Autodesk Inventor part; units mm, degrees
ref_plane "YZ Plane" through (0, 0, 0) normal (1, 0, 0) x (0, 1, 0)
ref_plane "XZ Plane" through (0, 0, 0) normal (0, 1, 0) x (-1, 0, 0)
ref_plane "XY Plane" through (0, 0, 0) normal (0, 0, 1) x (1, 0, 0)
sketch "Sketch1" plane through (0, 0, 0) normal (0, 0, 1) x (1, 0, 0)
  line L0 (-10.4918, 19.8361) -> (-50.4918, 19.8361)
  line L1 (-50.4918, 19.8361) -> (-50.4918, -15.1639)
  line L2 (-50.4918, -15.1639) -> (-10.4918, -15.1639)
  line L3 (-10.4918, -15.1639) -> (-10.4918, 19.8361)
  point P0 (0, 0)
  dimension "d0" = 40
  dimension "d1" = 35
extrude "Extrusion1" add sketch "Sketch1" along normal blind 5
sketch "Sketch2" plane through (0, 0, 0) normal (0, 0, -1) x (-1, 0, 0)
  line L0 (50.4918, 19.8361) -> (50.4918, -15.1639)
  line L1 (50.4918, 19.8361) -> (27.4918, 19.8361)
  line L2 (27.4918, 19.8361) -> (27.4918, 14.8361)
  line L3 (27.4918, 14.8361) -> (50.4918, 14.8361)
  line L4 (50.4918, 14.8361) -> (50.4918, 19.8361)
  point P0 (0, 0)
  point P1 (50.4918, 14.8361)
  dimension "d4" = 23
  dimension "d5" = 5
extrude "Extrusion2" add sketch "Sketch2" along normal blind 20
sketch "Sketch3" plane through (0, 0, 0) normal (0, 0, -1) x (-1, 0, 0)
  line L0 (27.4918, 14.8361) -> (50.4918, 14.8361)
  line L1 (50.4918, 19.8361) -> (50.4918, -15.1639)
  line L2 (50.4918, 15.8361) -> (47.4918, 15.8361)
  line L3 (47.4918, 15.8361) -> (47.4918, -4.1639)
  line L4 (47.4918, -4.1639) -> (50.4918, -4.1639)
  line L5 (50.4918, -4.1639) -> (50.4918, 15.8361)
  point P0 (0, 0)
  point P1 (47.4918, 14.8361)
  dimension "d8" = 20
  dimension "d9" = 3
extrude "Extrusion3" add sketch "Sketch3" along normal blind 20 contours L0 L1 L4 L3
sketch "Sketch4" plane through (-27.4918, 14.8361, -20) normal (0, -1, 0) x (1, 0, 0)
  circle A0 centre (-10, 10) radius 8
  line L0 (0, 0) -> (-20, 0)
  line L1 (0, 20) -> (0, 0)
  circle A1 centre (-2, 2) radius 1
  circle A2 centre (-18, 2) radius 1
  circle A3 centre (-18, 18) radius 1
  circle A4 centre (-2, 18) radius 1
  point P0 (27.4918, 20)
  dimension "d12" = 16
  dimension "d13" = 10
  dimension "d14" = 10
  dimension "d15" = 2
  dimension "d16" = 2
  dimension "d17" = 2
  dimension "d18" = 2
  dimension "d19" = 8
  dimension "d20" = 8
  dimension "d21" = 8
  dimension "d22" = 8
  dimension "d23" = 8
  dimension "d24" = 8
  dimension "d25" = 8
  dimension "d26" = 8
extrude "Extrusion4" cut sketch "Sketch4" against normal through all
fillet "Fillet1" radius 1.5 1 edges at (-27.4918, 17.3361, -20)
sketch "Sketch5" plane through (-47.4918, -4.1639, 0) normal (1, 0, 0) x (0, 0, -1)
  line L0 (20, 19) -> (20, 0)
  line L1 (0, 0) -> (20, 0)
  line L2 (20, 19) -> (0, 0)
  line L3 (0, 0) -> (20, 0)
  line L4 (20, 0) -> (20, 19)
  point P0 (0, 4.1639)
extrude "Extrusion5" cut sketch "Sketch5" against normal through all
fillet "Fillet2" radius 5 1 edges at (-48.9918, -4.1639, 0)
fillet "Fillet4" radius 2 1 edges at (-47.4918, 5.3361, 0)
sketch "Sketch6" plane through (0, 0, 5) normal (0, 0, 1) x (1, 0, 0)
  line L0 (-10.4918, 19.8361) -> (-50.4918, 19.8361)
  line L1 (-17.4918, 19.8361) -> (-43.4918, 19.8361)
  line L2 (-43.4918, 19.8361) -> (-43.4918, 14.8361)
  line L3 (-43.4918, 14.8361) -> (-17.4918, 14.8361)
  line L4 (-17.4918, 14.8361) -> (-17.4918, 19.8361)
  line L5 (-10.4918, -15.1639) -> (-10.4918, 19.8361)
  line L6 (-50.4918, 19.8361) -> (-50.4918, -15.1639)
  point P0 (0, 0)
  dimension "d39" = 5
  dimension "d40" = 7
  dimension "d41" = 7
extrude "Extrusion6" add sketch "Sketch6" along normal blind 46
chamfer "Chamfer2" distance 7 angle 45 2 edges at (-17.4918, 17.3361, 5) (-43.4918, 17.3361, 5)
sketch "Sketch7" plane through (-43.4918, 14.8361, 51) normal (0, -1, 0) x (1, 0, 0)
  circle A0 centre (13, -30.5) radius 1.5
  line L0 (-7, -46) -> (33, -46)
  line L1 (26, -39) -> (26, 0)
  point P0 (43.4918, -51)
  dimension "d47" = 3
  dimension "d48" = 15.5
  dimension "d49" = 13
extrude "Extrusion7" cut sketch "Sketch7" against normal through all
chamfer "Chamfer3" distance 1.8 angle 45 1 edges at (-31.9918, 19.8361, 20.5)
sketch "Sketch8" plane through (-27.4918, 19.8361, 0) normal (0, 1, 0) x (1, 0, 0)
  circle A0 centre (14, -2.5) radius 0.8
  circle A1 centre (6, -2.5) radius 0.8
  line L0 (17, 0) -> (0, 0)
  line L1 (17, 0) -> (17, -5)
  point P0 (27.4918, 0)
  dimension "d55" = 1.6
  dimension "d56" = 1.6
  dimension "d57" = 2.5
  dimension "d58" = 2.5
  dimension "d59" = 3
  dimension "d60" = 8
extrude "Extrusion8" cut sketch "Sketch8" against normal blind 10
chamfer "Chamfer4" distance 0.8 angle 45 2 edges at (-14.2918, 9.8361, 2.5) (-22.2918, 9.8361, 2.5)
fillet "Fillet5" radius 1 2 edges at (-14.2918, 10.6356, 2.5) (-22.2918, 10.6356, 2.5)
sketch "Sketch9" plane through (-50.4918, -15.1639, 0) normal (0, -1, 0) x (1, 0, 0)
  line L0 (40, 0) -> (40, 5)
  line L1 (40, 0) -> (23, 0)
  line L2 (40, 5) -> (26, 5)
  line L3 (26, 5) -> (26, 0)
  line L4 (26, 0) -> (40, 0)
  line L5 (40, 0) -> (40, 5)
  point P0 (50.4918, 0)
  dimension "d67" = 14
extrude "Extrusion9" add sketch "Sketch9" along normal blind 15
sketch "Sketch10" plane through (0, 0, 0) normal (0, 0, -1) x (-1, 0, 0)
  circle A0 centre (17.4918, -25.1639) radius 0.8
  line L0 (10.4918, 19.8361) -> (10.4918, -30.1639)
  line L1 (24.4918, -30.1639) -> (10.4918, -30.1639)
  circle A1 centre (17.4918, -5.1639) radius 0.8
  circle A2 centre (17.4918, 14.8361) radius 0.8
  point P0 (0, 0)
  dimension "d70" = 1.6
  dimension "d71" = 7
  dimension "d72" = 5
  dimension "d75" = 20
extrude "Extrusion10" cut sketch "Sketch10" against normal through all
fillet "Fillet6" radius 3 2 edges at (-50.4918, -15.1639, 2.5) (-24.4918, -15.1639, 2.5)
sketch "Sketch11" plane through (0, 0, 0) normal (0, 0, -1) x (-1, 0, 0)
  circle A0 centre (38.4918, -10.1639) radius 1.5
  circle A1 centre (30.4918, -10.1639) radius 1.5
  circle A2 centre (30.4918, -1.1639) radius 1.5
  circle A3 centre (38.4918, -1.1639) radius 1.5
  circle A4 centre (38.4918, 7.8361) radius 1.5
  circle A5 centre (30.4918, 7.8361) radius 1.5
  line L0 (47.4918, -15.1639) -> (27.4918, -15.1639)
  line L1 (50.4918, -6.3105) -> (50.4918, -12.1639)
  circle A6 centre (22.4918, -10.1639) radius 1.5
  circle A7 centre (22.4918, -1.1639) radius 1.5
  circle A8 centre (22.4918, 7.8361) radius 1.5
  point P0 (0, 0)
  point P1 (37.4918, -15.1639)
  dimension "d89" = 3
  dimension "d90" = 3
  dimension "d91" = 3
  dimension "d92" = 3
  dimension "d93" = 3
  dimension "d94" = 3
  dimension "d95" = 5
  dimension "d96" = 5
  dimension "d97" = 8
  dimension "d98" = 12
  dimension "d99" = 12
  dimension "d100" = 12
  dimension "d101" = 9
  dimension "d102" = 9
  dimension "d103" = 9
  dimension "d104" = 8
  dimension "d105" = 9
  dimension "d106" = 8
  dimension "d109" = 8
  dimension "d110" = 3
  dimension "d111" = 5
  dimension "d112" = 9
  dimension "d113" = 9
  dimension "d114" = 3
  dimension "d115" = 3
  dimension "d116" = 8
  dimension "d117" = 8
extrude "Extrusion11" cut sketch "Sketch11" against normal through all
chamfer "Chamfer7" distance 1.9 angle 45 9 edges at (-20.9918, 7.8361, 0) (-20.9918, -1.1639, 0) (-20.9918, -10.1639, 0) (-28.9918, -10.1639, 0) (-28.9918, -1.1639, 0) (-28.9918, 7.8361, 0) (-36.9918, 7.8361, 0) (-36.9918, -1.1639, 0) (-36.9918, -10.1639, 0)
sketch "Sketch12" plane through (-27.4918, 19.8361, 0) normal (0, 1, 0) x (1, 0, 0)
  circle A0 centre (2, -34) radius 1.5
  circle A1 centre (2, -47) radius 1.5
  circle A2 centre (-9, -34) radius 1.5
  circle A3 centre (-9, -47) radius 1.5
  line L0 (10, -51) -> (-16, -51)
  line L1 (10, -12) -> (10, -51)
  line L2 (-16, -12) -> (-16, -51)
  point P0 (27.4918, 0)
  dimension "d121" = 3
  dimension "d122" = 3
  dimension "d123" = 3
  dimension "d124" = 3
  dimension "d125" = 17
  dimension "d126" = 17
  dimension "d127" = 8
  dimension "d128" = 8
  dimension "d129" = 7
  dimension "d130" = 7
  dimension "d131" = 4
  dimension "d132" = 4
extrude "Extrusion12" cut sketch "Sketch12" against normal through all
fillet "Fillet7" radius 3 1 edges at (-27.4918, 17.3361, 0)
properties part number "Motor_holder_R" material "ABS Plastic"
The listing builds one solid part. Answer for the finished solid, in the listing's coordinates (mm). A direction names the side the tool comes from. Give positions to 0.01 mm unless a question says otherwise; leave off trailing zeros. Order: outer loops, then holes, each group sorted by start corner. A loop starts at its lowest first (then second) coordinate and runs counter-clockwise, first axis right, second up. Notation, with made-up numbers: (-35, 44.5) - (6, 44.5) arc R26 cw to (6, 77.5) - close; hole circle Ø9 at (57, 56.5). An arc over 180 degrees is marked (long way). Answer as CSV lines item,"result".
Q1. A cutting plane is placed at A-A, the plane z = 20.5. Determine the outline of the cut face in (x, y), and give its area (3 significant figures).
Answer key:
outline,"(-43.49, 14.84) - (-31.99, 14.84) - (-31.99, 18.04) - (-33.79, 19.84) - (-43.49, 19.84) - close; (-28.99, 14.84) - (-18.29, 14.84) arc R0.8 cw to (-17.49, 15.64) - (-17.49, 19.84) - (-27.19, 19.84) - (-28.99, 18.04) - close"
area,"111 mm^2"
Q2. A cutting plane is placed at C-C, the plane y = 3.5. Determine the outline of the cut face in (x, z).
Answer key:
outline,"(-50.49, -8.07) - (-47.49, -8.07) - (-47.49, -2) arc R2 cw to (-45.49, 0) - (-10.49, 0) - (-10.49, 5) - (-50.49, 5) - close"
Q3. Each of these flat-tipped pins is pushed along its axis until it touches: pin 1 Ø3.5 at (x, y) = (-38.49, -1.16) entering from +Z; pin 2 Ø12 at (x, y) = (-22.5, -8.5) entering from -Z; pin 3 Ø3 at (x, z) = (-13, 7.5) entering from -Y; pin 4 Ø12 at (x, z) = (-17, 23) entering from +Y. Where does it stop, or does it pass through?
Answer key:
pin 1,"stops at z = 5"
pin 2,"stops at z = 0"
pin 3,"stops at y = 14.84"
pin 4,"stops at y = 19.84"
Q4. A cutting plane is placed at D-D, the plane z = 38.5. Determine the outline of the cut face in (x, y).
Answer key:
outline,"(-43.49, 14.84) - (-18.29, 14.84) arc R0.8 cw to (-17.49, 15.64) - (-17.49, 19.84) - (-43.49, 19.84) - close"
Q5. A cutting plane is placed at B-B, the plane z = 47. Determine the outline of the cut face in (x, y).
Answer key:
outline,"(-43.49, 14.84) - (-37.99, 14.84) - (-37.99, 19.84) - (-43.49, 19.84) - close; (-34.99, 14.84) - (-26.99, 14.84) - (-26.99, 19.84) - (-34.99, 19.84) - close; (-23.99, 14.84) - (-18.29, 14.84) arc R0.8 cw to (-17.49, 15.64) - (-17.49, 19.84) - (-23.99, 19.84) - close"
Q6. Determine the mould class of faces 6 (the face through (-23.99, 7.22, 1.78)), 7 (the face through (-14.08, 15.5, 1.96)), 8 (the face through (-24.492, -24, 3)) for opening direction Z: pulls with the +Z half, pulls with the -Z half, needs draft (parallel to the pull), parting line crosses it, or undercut.
Answer key:
face 6,"pulls with the -Z half"
face 7,"undercut"
face 8,"needs draft"
Q7. Straight lines are drawn through the part: L1, parallel to X at y = 17.75, z = 34; L2, parallel to Y at x = -37, z = 37.5; L3, parallel to Z at x = -14, y = -6. For each, find the intervals that lie inside material, in ascending order.
Answer key:
L1,"x = -43.49 to -37.99, -34.99 to -26.99, -23.99 to -17.49"
L2,"y = 14.84 to 19.84"
L3,"z = 0 to 5"
Q8. Which of the six approach directions +Z, -Z, +X, -X, +Y, -Y give full straight-line access (tool end or side, diameter ignored) to faces 1 (the face through (-31, 14.836, -5)), 2 (the face through (-27.492, 17, -11)), 3 (the face through (-14.04, 17.3, 8.55)), 4 (the face through (-16.9, -5.7, 2.5)), 5 (the face through (-43.492, 17, 31))?
Answer key:
face 1,"-Z, +X, -Y"
face 2,"-Z, +X, +Y, -Y"
face 3,"+Z, +X, +Y, -Y"
face 4,"+Z, -Z"
face 5,"+Z, -X, +Y, -Y"
